Source: CAD feature listing. Evaluate the final solid. Frame: model axes, mm. A direction names the side the tool comes from. Give positions to 0.01 mm unless a question says otherwise; leave off trailing zeros. Write each loop counter-clockwise with the first axis right and the second up, starting at its lowest first coordinate (ties: lowest second). Pieces come first, ordered by that corner, then holes.
```python
from build123d import *

# Parameters (mm, degrees)
F2_R     = 25.4
F2_R_2   = 1.7145
F4_DEPTH = 12.7
F0_R     = 31.75
F0_R_2   = 1.7145
F5_DEPTH = 12.7
F6_R     = 1.7145
F7_DEPTH = 3.81
F8_SIZE2 = 12.69999
F8_SIZE  = 12.69999


# Not quite as in the source:
# - a fillet or chamfer is up to 0.001 mm smaller than in the source, because OpenCascade refuses the exact size


with BuildPart() as f4:
    # F2 (on offset) → F4 (new body)
    with BuildSketch(Plane.XY.offset(12.7)):
        with Locations((-31.75, 31.75)):
            Circle(F2_R)
        with Locations((-31.75, 31.75)):
            Circle(F2_R_2, mode=Mode.SUBTRACT)
    extrude(amount=-F4_DEPTH)

    # F0 (on Top) → F5 (join)
    with BuildSketch(Plane.XY):
        with Locations((-31.75, 31.75)):
            Circle(F0_R)
        with Locations((-31.75, 31.75)):
            Circle(F0_R_2, mode=Mode.SUBTRACT)
    extrude(amount=F5_DEPTH)

    # F6 (on face) → F7 (cut)
    with BuildSketch(Plane.XY.offset(12.7)):
        Polygon((-27.813, 29.4769719902), (-27.813, 34.0230280098), (-31.75, 36.2960560196), (-35.687, 34.0230280098), (-35.687, 29.4769719902), (-31.75, 27.2039439804), align=None)
        with Locations((-31.75, 31.75)):
            Circle(F6_R, mode=Mode.SUBTRACT)
    extrude(amount=-F7_DEPTH, mode=Mode.SUBTRACT)

    # F8 (size 12.7 and 12.7 in the source; OpenCascade refuses exactly that, so slightly less here)
    f8_edges = [f4.edges().sort_by_distance(p)[0] for p in [
        (-63.5, 31.75, 12.7),
    ]]
    chamfer(f8_edges, length=F8_SIZE, length2=F8_SIZE2)


solid = f4.part
```
1. Pin query (flat end, axial travel): P1, Ø3, axis at y = 44.5, z = 8.5, coming from the -X side; P2, Ø4, axis at x = -19.5, y = 8, coming from the -Z side; P3, Ø4, axis at y = 31, z = 11, coming from the -X side; P4, Ø4, axis at y = 32, z = 11, coming from the +X side. Return the tip coordinate at first contact, or that it passes through.
2. Line query: probe 1 along X at (y, z) = (34, 12.25); probe 2 along Y at (x, z) = (-31.75, 3.25); probe 3 along Y at (x, z) = (-31.75, 2). Output: solid intervals per line, ascending.
3. Section query C-C (z = 6). Return loops of the section in (x, y).
4. Access query for faces 4 (the flat face through (-32, 25, 0)), 5 (the flat face through (-34, 32, 8.89)). Directions: +Z, -Z, +X, -X, +Y, -Y. A direction counts if a zero-diameter tool reaches every point of the face in a straight line with its end or side. Return the directions, or none.
5. Pull-direction query (X, two-part tool) for faces 1 (the flat face through (-36, 32, 12.7)), 2 (the conical face through (-47.36, 19.78, 12.08)), 3 (the cylindrical face through (-33.111, 30.707, 4.507)); classes: pulls with the +X half, pulls with the -X half, needs draft (parallel to the pull), parting line crosses it, or undercut.
6. Section query B-B (z = 2.5). Return loops of the section in (x, y), plus the area to 3 significant figures.
The answers:
1. P1: stops at x = -53.17
1. P2: stops at z = 0
1. P3: stops at x = -54.49
1. P4: stops at x = -9
2. probe 1: x = -51.12 to -35.69, -27.81 to -12.38
2. probe 2: y = 3.25 to 30.04, 33.46 to 60.25
2. probe 3: y = 2 to 30.04, 33.46 to 61.5
3. outline: circle Ø51.5 at (-31.75, 31.75); hole circle Ø3.43 at (-31.75, 31.75)
4. face 4: -Z, +X, -X, +Y, -Y
4. face 5: +Z
5. face 1: needs draft
5. face 2: parting line crosses it
5. face 3: undercut
6. outline: circle Ø58.5 at (-31.75, 31.75); hole circle Ø3.43 at (-31.75, 31.75)
6. area: 2,680 mm2
